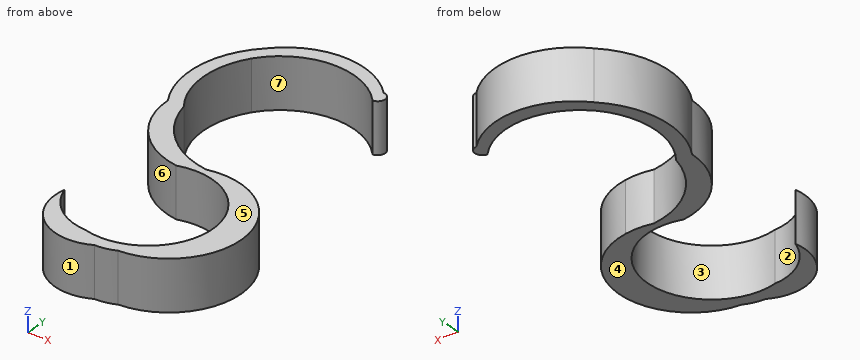
from build123d import *

# Parameters (mm, degrees)
F1_DEPTH = 12.7


with BuildPart() as f1:
    # F0 (on Top) → F1 (new body)
    with BuildSketch(Plane.XY):
        with BuildLine():
            ThreePointArc((6.969989, -33.608161), (3.356066, -32.709161), (0, -31.095017))
            ThreePointArc((0, -31.095017), (-7.898027, -28.011691), (-12.548544, -20.922374))
            ThreePointArc((-12.548544, -20.922374), (-8.221346, -33.529552), (5.044016, -34.831756))
            ThreePointArc((5.044016, -34.831756), (6.035373, -34.264614), (6.969989, -33.608161))
        make_face()
        with BuildLine():
            ThreePointArc((0, 0), (20.620834, -15.547508), (0, -31.095017))
            ThreePointArc((0, -31.095017), (3.356066, -32.709161), (6.969989, -33.608161))
            ThreePointArc((6.969989, -33.608161), (8.584093, -33.765391), (10.205782, -33.778654))
            ThreePointArc((10.205782, -33.778654), (27.738488, -16.878906), (12.85268, 2.393092))
            ThreePointArc((12.85268, 2.393092), (9.320558, 2.059582), (5.78111, 2.303358))
            ThreePointArc((5.78111, 2.303358), (2.791616, 1.400004), (0, 0))
        make_face()
        with BuildLine():
            ThreePointArc((-16.308, 19.54706), (-11.822589, 6.712847), (0, 0))
            ThreePointArc((0, 0), (2.791616, 1.400004), (5.78111, 2.303358))
            ThreePointArc((5.78111, 2.303358), (-5.99092, 8.071132), (-12.327401, 19.54706))
            ThreePointArc((-12.327401, 19.54706), (-15.987157, 31.157143), (-12.327401, 42.767227))
            ThreePointArc((-12.327401, 42.767227), (2.110379, 50.457564), (17.084811, 43.872949))
            ThreePointArc((17.084811, 43.872949), (18.857216, 45.752674), (17.084811, 47.6324))
            ThreePointArc((17.084811, 47.6324), (2.378705, 54.134652), (-12.327401, 47.6324))
            ThreePointArc((-12.327401, 47.6324), (-19.279128, 34.292925), (-16.308, 19.54706))
        make_face()
        with BuildLine():
            ThreePointArc((10.205782, -33.778654), (8.584093, -33.765391), (6.969989, -33.608161))
            ThreePointArc((6.969989, -33.608161), (6.035373, -34.264614), (5.044016, -34.831756))
            ThreePointArc((5.044016, -34.831756), (7.683397, -34.591928), (10.205782, -33.778654))
        make_face()
        with BuildLine():
            ThreePointArc((12.85268, 2.393092), (9.312505, 2.694176), (5.78111, 2.303358))
            ThreePointArc((5.78111, 2.303358), (9.320558, 2.059582), (12.85268, 2.393092))
        make_face()
    extrude(amount=F1_DEPTH)


solid = f1.part
Read the model definition and answer for the solid it produces. Units are mm, in the model's axes. Face numbers are marked on the shaded views. A direction names the side the tool comes from. Round coordinates to 2 decimals unless told otherwise and drop trailing zeros. Write each loop counter-clockwise with the first axis right and the second up, starting at its lowest first coordinate (ties: lowest second). Pieces come first, ordered by that corner, then holes. Notation, with made-up numbers: (-28, -29.75) - (-5, -29.75) arc R8 cw to (-5, -14.75) - close; hole circle Ø5 at (-31.5, 68). An arc over 180 degrees is marked (long way). Use a Markdown table: item, result.
(1) Each of these flat-tipped pins is pushed along its axis until it touches: pin 1 Ø5 at (x, z) = (-13, 3) entering from -Y; pin 2 Ø2 at (x, z) = (21.5, 4) entering from -Y; pin 3 Ø1 at (x, z) = (13, 8.5) entering from -Y. Where does it stop, or does it pass through?
Reported:
| item | result |
|---|---|
| pin 1 | y = -31.17 |
| pin 2 | y = -30.13 |
| pin 3 | y = -33.55 |
(2) The part is cut by section A-A (x = 15). Write down the section's boundary in (y, z), then the cut area to 3 significant figures.
Reported:
| item | result |
|---|---|
| outline | (-32.96, 0) - (-27.8, 0) - (-27.8, 12.7) - (-32.96, 12.7) - close; (-3.29, 0) - (1.86, 0) - (1.86, 12.7) - (-3.29, 12.7) - close; (45.97, 0) - (49.61, 0) - (49.61, 12.7) - (45.97, 12.7) - close |
| area | 177 mm2 |
(3) Straight lines are drawn through the part: line 1 along Y through (x, z) = (3.5, 2); line 2 along Y through (x, z) = (-1.5, 9.25); line 3 along X through (y, z) = (48, 1.5). For each, find the intervals that lie inside material, in ascending order. Write a range as [from, to].
Reported:
| item | result |
|---|---|
| line 1 | [-35.49, -31.69], [0.6, 2.77], [50.46, 54.1] |
| line 2 | [-36.15, -30.92], [0.3, 4.78], [49.97, 53.75] |
| line 3 | [-11.98, -6.48], [12.11, 16.74] |
(4) The part is cut by section C-C (x = -14). Write down the section's boundary in (y, z), then the cut area to 3 significant figures.
Reported:
| item | result |
|---|---|
| outline | (9.93, 0) - (22.41, 0) - (22.41, 12.7) - (9.93, 12.7) - close; (39.9, 0) - (45.9, 0) - (45.9, 12.7) - (39.9, 12.7) - close |
| area | 235 mm2 |
(5) The mould has two halves that part along X. Classify the marked faces 1, 2, 3 and 4: released by +X, released by -X, zero draft, split by the parting line, or undercut.
Reported:
| item | result |
|---|---|
| face 1 | split by the parting line |
| face 2 | undercut |
| face 3 | undercut |
| face 4 | zero draft |
(6) The part is cut by section B-B (z = 10.5). Write down the section's boundary in (x, y), then the cut area to 3 significant figures.
Reported:
| item | result |
|---|---|
| outline | (-16.31, 19.55) arc R19.34 ccw to (0, 0) arc R16.17 cw (long way) to (0, -31.1) arc R13.94 cw to (-12.55, -20.92) arc R12.33 ccw to (5.04, -34.83) arc R12 ccw to (10.21, -33.78) arc R18.24 ccw to (12.85, 2.39) arc R18.24 ccw to (5.78, 2.3) arc R21.8 cw to (-12.33, 19.55) arc R20.25 cw to (-12.33, 42.77) arc R18.73 cw to (17.08, 43.87) arc R1.88 ccw to (17.08, 47.63) arc R19.88 ccw to (-12.33, 47.63) arc R22.58 ccw to start |
| area | 733 mm2 |
(7) The part is cut by section D-D (x = 2). Write down the section's boundary in (y, z), then the cut area to 3 significant figures.
Reported:
| item | result |
|---|---|
| outline | (-35.91, 0) - (-31.53, 0) - (-31.53, 12.7) - (-35.91, 12.7) - close; (0.44, 0) - (3.23, 0) - (3.23, 12.7) - (0.44, 12.7) - close; (50.45, 0) - (54.13, 0) - (54.13, 12.7) - (50.45, 12.7) - close |
| area | 138 mm2 |
(8) Which of the six approach directions +Z, -Z, +X, -X, +Y, -Y give full straight-line access (tool end or side, diameter ignored) to the marked faces 5, 6 and 7?
Reported:
| item | result |
|---|---|
| face 5 | +Z, +X, -X, +Y, -Y |
| face 6 | +Z, -Z, -X |
| face 7 | +Z, -Z |
